CAD build for the part. Positions are in the model's coordinates, mm. A direction names the side the tool comes from. Give positions to 0.01 mm unless a question says otherwise; leave off trailing zeros. Loops run counter-clockwise (first coordinate to the right, second up) from the corner with the lowest first, then second, coordinate; pieces in that order, holes last. Notation, with made-up numbers: M 17.25,-21.5 L 67.25,-21.5 A22 cw 67.25,-1.5 Z; hole C 75,67.25 d8. An arc over 180 degrees is marked long. One line per question, with ' | ' between items.
```python
from build123d import *

# Parameters (mm, degrees)
SKETCH1_W           = 10.1
SKETCH1_H           = 10.1
BOSS_EXTRUDE1_DEPTH = 5.4
SKETCH2_W           = 1
SKETCH2_H           = 1
BOSS_EXTRUDE2_DEPTH = 1
SKETCH3_W           = 2.5
SKETCH3_H           = 0.8
BOSS_EXTRUDE3_DEPTH = 0.5


with BuildPart() as part:
    # Sketch1 → Boss-Extrude1 (new body)
    with BuildSketch(Plane(origin=(0, 0, 0), x_dir=(1, 0, 0), z_dir=(0, 1, 0))):
        Rectangle(SKETCH1_W, SKETCH1_H)
    extrude(amount=BOSS_EXTRUDE1_DEPTH)

    # Sketch2 → Boss-Extrude2 (add)
    with BuildSketch(Plane(origin=(0, 5.4, 0), x_dir=(1, 0, 0), z_dir=(0, 1, 0))):
        with BuildLine():
            ThreePointArc((0.5, 2.958039892), (0, 3), (-0.5, 2.958039892))
            Line((-0.5, 2.958039892), (-0.5, 2.193741097))
            ThreePointArc((-0.5, 2.193741097), (0, 2.25), (0.5, 2.193741097))
            Line((0.5, 2.193741097), (0.5, 2.958039892))
        make_face()
        with BuildLine():
            Line((-0.5, -2.193741097), (-0.5, -2.958039892))
            ThreePointArc((-0.5, -2.958039892), (0, -3), (0.5, -2.958039892))
            Line((0.5, -2.958039892), (0.5, -2.193741097))
            ThreePointArc((0.5, -2.193741097), (0, -2.25), (-0.5, -2.193741097))
        make_face()
        with BuildLine():
            ThreePointArc((0.5, 2.193741097), (0, 2.25), (-0.5, 2.193741097))
            Line((-0.5, 2.193741097), (-0.5, 0.5))
            Line((-0.5, 0.5), (0.5, 0.5))
            Line((0.5, 0.5), (0.5, 2.193741097))
        make_face()
        with BuildLine():
            Line((-0.5, 0.5), (-0.5, 2.193741097))
            ThreePointArc((-0.5, 2.193741097), (-1.590990258, 1.590990258), (-2.193741097, 0.5))
            Line((-2.193741097, 0.5), (-0.5, 0.5))
        make_face()
        with BuildLine():
            Line((-0.5, -0.5), (-0.5, 0.5))
            Line((-0.5, 0.5), (-2.193741097, 0.5))
            ThreePointArc((-2.193741097, 0.5), (-2.25, 0), (-2.193741097, -0.5))
            Line((-2.193741097, -0.5), (-0.5, -0.5))
        make_face()
        with BuildLine():
            Line((-2.193741097, 0.5), (-2.958039892, 0.5))
            ThreePointArc((-2.958039892, 0.5), (-3, 0), (-2.958039892, -0.5))
            Line((-2.958039892, -0.5), (-2.193741097, -0.5))
            ThreePointArc((-2.193741097, -0.5), (-2.25, 0), (-2.193741097, 0.5))
        make_face()
        with BuildLine():
            ThreePointArc((3, 0), (2.989491568, 0.250878781), (2.958039892, 0.5))
            Line((2.958039892, 0.5), (2.193741097, 0.5))
            ThreePointArc((2.193741097, 0.5), (2.235891038, 0.251577555), (2.25, 0))
            ThreePointArc((2.25, 0), (2.235891038, -0.251577555), (2.193741097, -0.5))
            Line((2.193741097, -0.5), (2.958039892, -0.5))
            ThreePointArc((2.958039892, -0.5), (2.989491568, -0.250878781), (3, 0))
        make_face()
        with BuildLine():
            Line((0.5, -0.5), (-0.5, -0.5))
            Line((-0.5, -0.5), (-0.5, -2.193741097))
            ThreePointArc((-0.5, -2.193741097), (0, -2.25), (0.5, -2.193741097))
            Line((0.5, -2.193741097), (0.5, -0.5))
        make_face()
        Rectangle(SKETCH2_W, SKETCH2_H)
        with BuildLine():
            Line((2.193741097, 0.5), (0.5, 0.5))
            Line((0.5, 0.5), (0.5, -0.5))
            Line((0.5, -0.5), (2.193741097, -0.5))
            ThreePointArc((2.193741097, -0.5), (2.235891038, -0.251577555), (2.25, 0))
            ThreePointArc((2.25, 0), (2.235891038, 0.251577555), (2.193741097, 0.5))
        make_face()
        with BuildLine():
            ThreePointArc((2.193741097, 0.5), (1.590990258, 1.590990258), (0.5, 2.193741097))
            Line((0.5, 2.193741097), (0.5, 0.5))
            Line((0.5, 0.5), (2.193741097, 0.5))
        make_face()
        with BuildLine():
            Line((2.193741097, -0.5), (0.5, -0.5))
            Line((0.5, -0.5), (0.5, -2.193741097))
            ThreePointArc((0.5, -2.193741097), (1.590990258, -1.590990258), (2.193741097, -0.5))
        make_face()
        with BuildLine():
            Line((-0.5, -2.193741097), (-0.5, -0.5))
            Line((-0.5, -0.5), (-2.193741097, -0.5))
            ThreePointArc((-2.193741097, -0.5), (-1.590990258, -1.590990258), (-0.5, -2.193741097))
        make_face()
    extrude(amount=BOSS_EXTRUDE2_DEPTH)

    # Sketch3 → Boss-Extrude3 (add)
    with BuildSketch(Plane.XZ):
        with Locations((-6.3, 3.81)):
            Rectangle(SKETCH3_W, SKETCH3_H)
        with Locations((6.3, 3.81)):
            Rectangle(SKETCH3_W, SKETCH3_H)
        with Locations((6.3, -3.81)):
            Rectangle(SKETCH3_W, SKETCH3_H)
        with Locations((-6.3, -3.81)):
            Rectangle(SKETCH3_W, SKETCH3_H)
    extrude(amount=-BOSS_EXTRUDE3_DEPTH)


solid = part.part
```
Item 1: Drop flat-ended pins along their axis: P1, Ø2.5, axis at y = 2, z = 1, coming from the -X side; P2, Ø0.6, axis at x = -6.5, y = 0, coming from the -Z side; P3, Ø5, axis at x = -2.5, z = 1.5, coming from the +Y side; P4, Ø0.6, axis at x = 5.5, y = 0.5, coming from the +Z side. Give the stop position or say it passes through.
Conclusion:
P1: x = -5.05 | P2: z = -4.21 | P3: y = 6.4 | P4: z = 4.21
Item 2: Saw through at B-B on z = -2.5. Give the cut face in (x, y).
Conclusion:
outline: M -5.05,0 L 5.05,0 L 5.05,5.4 L 0.5,5.4 L 0.5,6.4 L -0.5,6.4 L -0.5,5.4 L -5.05,5.4 Z
Item 3: 3-axis set-ups, long thin cutter, end or side, ignore diameter. For faces 1 (the cylindrical face through (1.6, 5.89, -1.58)), 2 (the cylindrical face through (-1.58, 5.89, -1.6)), 3 (the cylindrical face through (0, 6, -3)): which of +Z, -Z, +X, -X, +Y, -Y reach the whole face in a straight line?
Conclusion:
face 1: -Z, +X, +Y | face 2: -Z, -X, +Y | face 3: -Z, +Y
Item 4: Saw through at D-D on y = 2. Give the cut face in (x, z).
Conclusion:
outline: M -5.05,-5.05 L 5.05,-5.05 L 5.05,5.05 L -5.05,5.05 Z
Item 5: Saw through at C-C on x = 1.5. Give the cut face in (y, z).
Conclusion:
outline: M 0,-5.05 L 5.4,-5.05 L 5.4,-1.68 L 6.4,-1.68 L 6.4,1.68 L 5.4,1.68 L 5.4,5.05 L 0,5.05 Z
Item 6: Saw through at A-A on x = 6.75. Give the cut face in (y, z), and give its area (3 significant figures).
Conclusion:
outline: M 0,-4.21 L 0.5,-4.21 L 0.5,-3.41 L 0,-3.41 Z; M 0,3.41 L 0.5,3.41 L 0.5,4.21 L 0,4.21 Z | area: 0.800 mm²
Item 7: Drill centre lines: line 1 along X through (y, z) = (4.25, 4.75); line 2 along Y through (x, z) = (4.25, -2.25); line 3 along Z through (x, y) = (1.5, 5.5). Where is each one in solid material? Low to high. Write a range as [from, to].
Conclusion:
line 1: [-5.05, 5.05] | line 2: [0, 5.4] | line 3: [-1.68, 1.68]
